Source: CAD feature listing. Evaluate the final solid. Frame: model axes, mm. A direction names the side the tool comes from. Coordinates: 2 decimals unless noted, no trailing zeros. Loops run counter-clockwise (first coordinate to the right, second up) from the corner with the lowest first, then second, coordinate; pieces in that order, holes last.
```python
from build123d import *

# Parameters (mm, degrees)
F1_DEPTH  = 4.7625
F2_R      = 3.96875
F3_DEPTH  = 20.32
F4_R      = 4.646824
F5_DEPTH  = 1.27
F6_R      = 9.525
F7_DEPTH  = 1.27
F8_R      = 8.115577
F8_R_2    = 5.810874
F9_DEPTH  = 0.127
F10_R     = 7.9375
F11_DEPTH = 6.35
F12_R     = 4.795683
F13_DEPTH = 1.905
F14_R     = 7.919715
F15_DEPTH = 0.635


with BuildPart() as f1:
    # F0 (on Front) → F1 (new body)
    with BuildSketch(Plane.XZ):
        Polygon((-3.70389, 6.328075), (-7.332219, -0.043625), (-3.628329, -6.3717), (3.70389, -6.328075), (7.332219, 0.043625), (3.628329, 6.3717), align=None)
    extrude(amount=F1_DEPTH)

    # F2 (on face) → F3 (join)
    with BuildSketch(Plane.XZ.offset(4.7625)):
        Circle(F2_R)
    extrude(amount=F3_DEPTH)

    # F4 (on face) → F5 (join)
    with BuildSketch(Plane.XZ.offset(4.7625)):
        with Locations((-0.133895, 0)):
            Circle(F4_R)
    extrude(amount=F5_DEPTH)

    # F6 (on face) → F7 (join)
    with BuildSketch(Plane.XZ.offset(6.0325)):
        Circle(F6_R)
    extrude(amount=F7_DEPTH)

    # F8 (on face) → F9 (cut)
    with BuildSketch(Plane(origin=(0, -6.0325, 0), x_dir=(-1, 0, 0), z_dir=(0, 1, 0))):
        Circle(F8_R)
        Circle(F8_R_2, mode=Mode.SUBTRACT)
    extrude(amount=-F9_DEPTH, mode=Mode.SUBTRACT)

    # F10 (on face) → F11 (join)
    with BuildSketch(Plane.XZ.offset(7.3025)):
        Circle(F10_R)
    extrude(amount=F11_DEPTH)

    # F12 (on face) → F13 (join)
    with BuildSketch(Plane.XZ.offset(13.6525)):
        Circle(F12_R)
    extrude(amount=F13_DEPTH)

    # F14 (on face) → F15 (join)
    with BuildSketch(Plane.XZ.offset(15.5575)):
        Circle(F14_R)
    extrude(amount=F15_DEPTH)

    # F16: F1 across face


with BuildPart() as f1_1:
    add(f1.part)
    add(f1.part.mirror(Plane.XZ.offset(25.0825)))


solid = f1_1.part
```
Q1. Section query A-A on y = -3. Return the cut outline in (x, z), then the cut area to 3 significant figures.
Q2. Material intervals for line 1 along Z through (x, y) = (0, -44.05) (3 decimals); line 2 along Y through (x, z) = (1.25, -6) (1 decimal); line 3 along Y through (x, z) = (4.75, -7), sorted ascending.
Q3. Reachability of faces 1 (the flat face through (5.49, -2.35, -3.19)), 2 (the flat face through (-4, -16.192, -2)), 3 (the flat face through (-5.49, -47.82, 3.19)), 4 (the flat face through (5.51, -47.82, 3.16)) from +Z, -Z, +X, -X, +Y, -Y: full face, straight path, thin tool, end or side. Return the list, or none.
Q4. Section query B-B on x = -6.5. Count the separate pieces of the cut face and the enclosed holes in it, then the cut area to 3 significant figures.
Q5. First-contact query: pin 1 Ø3 at (x, y) = (-1.5, -36) entering from -Z; pin 2 Ø3 at (x, y) = (7, -9) entering from -Z; pin 3 Ø3 at (x, y) = (-4.5, -22.5) entering from +Z. Flat tips, straight axial feed; report the tip coordinate or a pass-through.
Q6. Section query C-C on y = -18. Return the cut outline in (x, z), then the cut area to 3 significant figures.
Resolved:
1. outline: (-7.33, -0.04) - (-3.63, -6.37) - (3.7, -6.33) - (7.33, 0.04) - (3.63, 6.37) - (-3.7, 6.33) - close
1. area: 140 mm2
2. line 1: z = -9.525 to -8.116, -5.811 to 5.811, 8.116 to 9.525
2. line 2: y = -50.2 to -45.4, -44 to -36.5, -34.6 to -34, -16.2 to -15.6, -13.7 to -6.2, -4.8 to 0
2. line 3: y = -44.13 to -42.86, -7.3 to -6.03
3. face 1: -Z, +X, +Y
3. face 2: none
3. face 3: +Z, -X, -Y
3. face 4: +Z, +X, -Y
4. separate pieces: 6
4. enclosed holes: 0
4. area: 188 mm2
5. pin 1: stops at z = -7.94
5. pin 2: stops at z = -5.72
5. pin 3: stops at z = 2.6
6. outline: circle Ø7.94 at (0, 0)
6. area: 49.5 mm2
